Input: part model. Units: mm. Frame: model coordinates. A direction names the side the tool comes from. Give positions to 0.01 mm unless a question says otherwise; leave off trailing zeros. Loops run counter-clockwise (first coordinate to the right, second up) from the corner with the lowest first, then second, coordinate; pieces in that order, holes last. Notation, with made-up numbers: (29.25, -31) -> (51.25, -31) arc R24 ccw to (51.25, -2) -> close; hole circle Ø3 at (-38, 78). An arc over 180 degrees is marked (long way). Answer in a Markdown table with one row per item. Add a question column.
```python
from build123d import *

# Parameters (mm, degrees)
SKICA1_R                 = 1.5
P_IDAT_VYSUNUT_M1_DEPTH  = 8
SKICA2_R                 = 2.25
P_IDAT_VYSUNUT_M2_DEPTH  = 3.75
ODEBRAT_VYSUNUT_M1_DEPTH = 2.25
ZKOSEN_1_SIZE            = 0.25
ZKOSEN_2_SIZE            = 0.25


with BuildPart() as part:
    # Skica1 → Přidat vysunutím1 (new body)
    with BuildSketch(Plane(origin=(0, 0, 0), x_dir=(1, 0, 0), z_dir=(0, 1, 0))):
        with Locations(Location((0, 0, 0), (0, 0, 270))):
            Circle(SKICA1_R)
    extrude(amount=P_IDAT_VYSUNUT_M1_DEPTH)

    # Skica2 → Přidat vysunutím2 (add)
    with BuildSketch(Plane(origin=(0, 8, 0), x_dir=(1, 0, 0), z_dir=(0, 1, 0))):
        with Locations(Location((0, 0, 0), (0, 0, 270))):
            Circle(SKICA2_R)
    extrude(amount=P_IDAT_VYSUNUT_M2_DEPTH)

    # Skica3 → Odebrat vysunutím1 (cut)
    with BuildSketch(Plane(origin=(0, 11.75, 0), x_dir=(1, 0, 0), z_dir=(0, 1, 0))):
        Polygon((-1.074402598, -0.875019461), (0.220587783, -1.367969674), (1.294990381, -0.492950213), (1.074402598, 0.875019461), (-0.220587783, 1.367969674), (-1.294990381, 0.492950213), align=None)
    extrude(amount=-ODEBRAT_VYSUNUT_M1_DEPTH, mode=Mode.SUBTRACT)

    # Zkosení1
    zkosen_1_edges = [part.edges().sort_by_distance(p)[0] for p in [
        (0, 11.75, -2.25),
    ]]
    chamfer(zkosen_1_edges, length=ZKOSEN_1_SIZE)

    # Zkosení2
    zkosen_2_edges = [part.edges().sort_by_distance(p)[0] for p in [
        (0, 0, -1.5),
    ]]
    chamfer(zkosen_2_edges, length=ZKOSEN_2_SIZE)


solid = part.part
```
1) Section D-D on y = 1. Output: boundary loops of the cut face in (x, z), and give its area (3 significant figures).
2) Pull-direction query (X, two-part tool) for faces 1 (the face through (0, 9.5, 0)), 2 (the face through (1, 11.75, 1)), 3 (the face through (0.45, 4.07, 1.43)); classes: +X half, -X half, draft (parallel to the pull), parting line (faces both ways), or undercut.
3) Section A-A on y = 11. Output: boundary loops of the cut face in (x, z) (3 decimals).
4) Section C-C on x = 0. Output: boundary loops of the cut face in (y, z).
5) Pin query (flat end, axial travel): pin 1 (2 mm diameter, centred on x = 1.5, y = 3.5, fed in from +Z); pin 2 (2 mm diameter, centred on x = 0, z = 0, fed in from +Y). Return the tip coordinate at first contact, or that it passes through.
6) Material intervals for line 1 along Y through (x, z) = (1.6, 0.3); line 2 along Y through (x, z) = (-0.95, -0.45); line 3 along Z through (x, y) = (0.6, 10.5), sorted ascending.
7) Section B-B on z = 0. Output: boundary loops of the cut face in (x, y).
8) Reachability of faces 4 (the face through (0, 8, -2)), 5 (the face through (0, 0, 0)), 6 (the face through (0.75, 10.641, 0.937)) from +Z, -Z, +X, -X, +Y, -Y: full face, straight path, thin tool, end or side. Return the list, or none.
Working result:
| question | item | result |
|---|---|---|
| 1 | outline | circle Ø3 at (0, 0) |
| 1 | area | 7.07 mm2 |
| 2 | face 1 | undercut |
| 2 | face 2 | draft |
| 2 | face 3 | parting line |
| 3 | outline | circle Ø4.5 at (0, 0); hole (-1.295, -0.493) -> (-0.221, -1.368) -> (1.074, -0.875) -> (1.295, 0.493) -> (0.221, 1.368) -> (-1.074, 0.875) -> close |
| 4 | outline | (0, -1.25) -> (0.25, -1.5) -> (8, -1.5) -> (8, -2.25) -> (11.5, -2.25) -> (11.75, -2) -> (11.75, -1.28) -> (9.5, -1.28) -> (9.5, 1.28) -> (11.75, 1.28) -> (11.75, 2) -> (11.5, 2.25) -> (8, 2.25) -> (8, 1.5) -> (0.25, 1.5) -> (0, 1.25) -> close |
| 5 | pin 1 | stops at z = 1.41 |
| 5 | pin 2 | stops at y = 9.5 |
| 6 | line 1 | y = 8 to 11.75 |
| 6 | line 2 | y = 0 to 9.5 |
| 6 | line 3 | z = -2.17 to -1.06, 1.06 to 2.17 |
| 7 | outline | (-2.25, 8) -> (-1.5, 8) -> (-1.5, 0.25) -> (-1.25, 0) -> (1.25, 0) -> (1.5, 0.25) -> (1.5, 8) -> (2.25, 8) -> (2.25, 11.5) -> (2, 11.75) -> (1.22, 11.75) -> (1.22, 9.5) -> (-1.22, 9.5) -> (-1.22, 11.75) -> (-2, 11.75) -> (-2.25, 11.5) -> close |
| 8 | face 4 | -Y |
| 8 | face 5 | +Z, -Z, +X, -X, -Y |
| 8 | face 6 | +Y |
